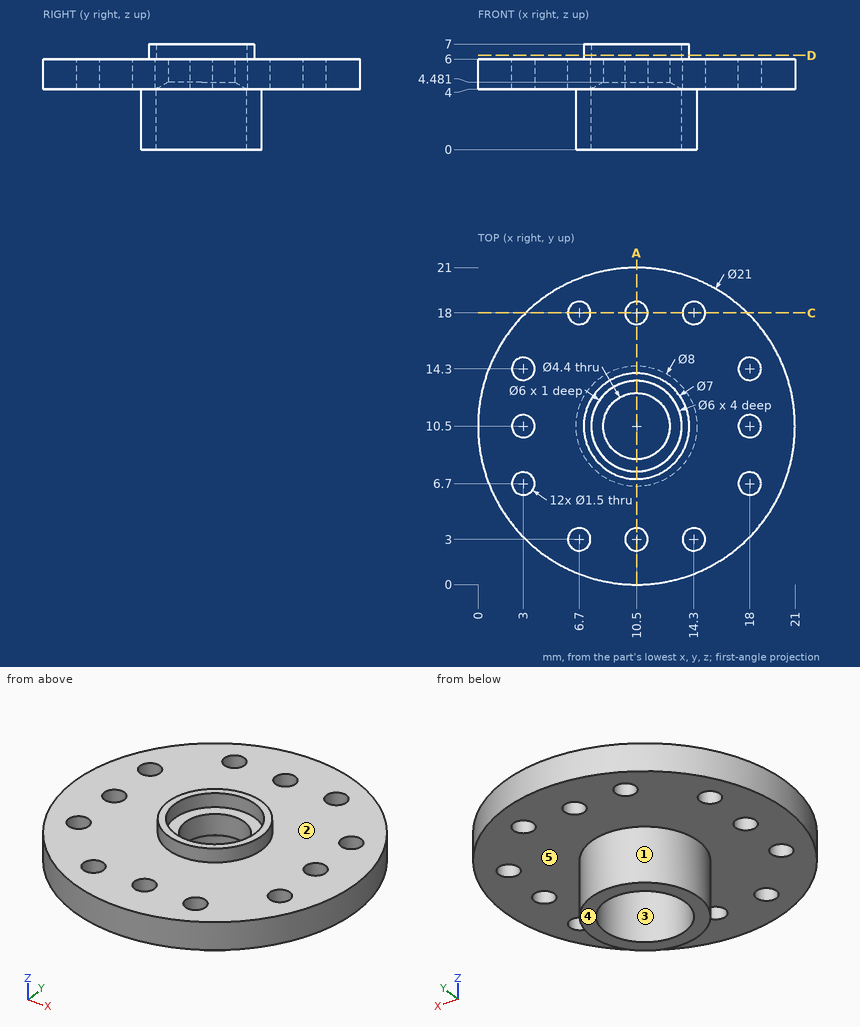
Geometry: see drawing. Coordinates: mm, zero at the bounding-box minimum. A direction names the side the tool comes from. Round coordinates to 2 decimals unless told otherwise and drop trailing zeros. Order: outer loops, then holes, each group sorted by start corner. A loop starts at its lowest first (then second) coordinate and runs counter-clockwise, first axis right, second up. Notation, with made-up numbers: (22, -7.5) - (59, -7.5) arc R29 cw to (59, 26.5) - close; hole circle Ø2 at (-21, 7.5). An arc over 180 degrees is marked (long way). One line per question, with ' | ' between items. Start each with the question number.
1) Set-up query: the marked faces 4 and 5. Return all of +Z, -Z, +X, -X, +Y, -Y with unobstructed straight access to the full face (end or side cutting, diameter ignored); none if empty.
2) Cut plane C-C, the plane y = 18. Return the cut outline in (x, z), then the cut area to 3 significant figures.
3) Cut plane A-A, the plane x = 10.5. Give the number of separate pieces and of enclosed holes in the cut face.
4) Ray query, probe 1 along Y at (x, z) = (3, 4.6); probe 2 along Y at (x, z) = (10.5, 6.5); probe 3 along Z at (x, y) = (13, 16.25). Return the intervals inside material, ascending.
5) Pull-direction query (X, two-part tool) for the marked faces 1, 2 and 3; classes: +X half, -X half, draft (parallel to the pull), parting line (faces both ways), or undercut.
6) Cut plane D-D, the plane z = 6.25. Return the cut outline in (x, y), then the cut area to 3 significant figures.
7) Contact query for flat-ended pins moving along their axis: P1, Ø2.5, axis at x = 3, y = 6.7, coming from the -Z side; P2, Ø0.9, axis at x = 10.5, y = 18, coming from the +Z side; P3, Ø2.5, axis at x = 6.7, y = 3, coming from the +Z side; P4, Ø2, axis at x = 3, z = 4.5, coming from the -Y side. Output: stop coordinate, or through.
Worked out:
1) face 4: -Z, +X, -X, +Y, -Y | face 5: -Z
2) outline: (3.15, 4) - (5.95, 4) - (5.95, 6) - (3.15, 6) - close; (7.45, 4) - (9.75, 4) - (9.75, 6) - (7.45, 6) - close; (11.25, 4) - (13.55, 4) - (13.55, 6) - (11.25, 6) - close; (15.05, 4) - (17.85, 4) - (17.85, 6) - (15.05, 6) - close | area: 20.4 mm^2
3) separate pieces: 4 | enclosed holes: 0
4) probe 1: y = 3.15 to 5.95, 7.45 to 9.75, 11.25 to 13.55, 15.05 to 17.85 | probe 2: y = 7 to 7.5, 13.5 to 14 | probe 3: z = 4 to 6
5) face 1: parting line | face 2: draft | face 3: undercut
6) outline: circle Ø7 at (10.5, 10.5); hole circle Ø6 at (10.5, 10.5) | area: 10.2 mm^2
7) P1: stops at z = 4 | P2: passes through | P3: stops at z = 6 | P4: stops at y = 2.25
